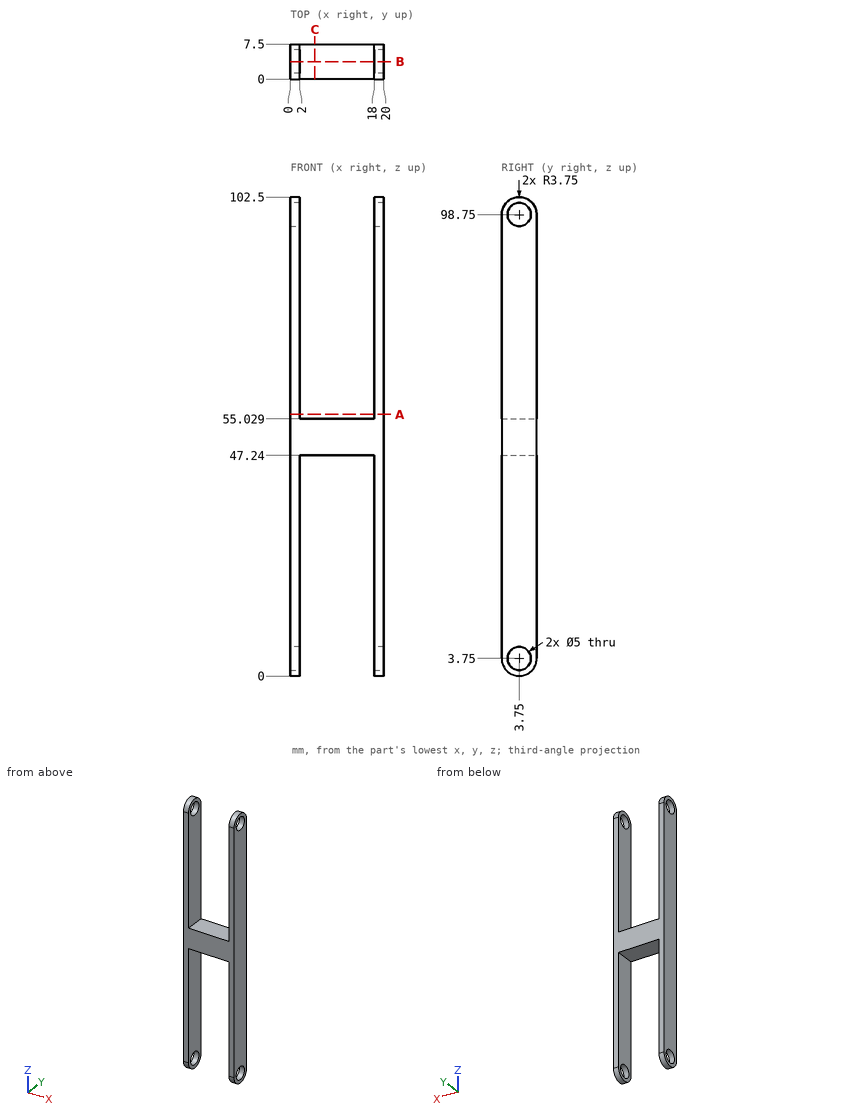
Study the drawing (mm; zero at the part's minimum x, y, z) and answer. Round coordinates to 2 decimals unless told otherwise and drop trailing zeros. Write each loop counter-clockwise with the first axis right and the second up, starting at its lowest first coordinate (ties: lowest second). Pieces come first, ordered by that corner, then holes.
Q1. Find section A-A on z = 56. Determine the outline of the cut face in (x, y).
Values:
outline: (0, 0) - (2, 0) - (2, 7.5) - (0, 7.5) - close; (18, 0) - (20, 0) - (20, 7.5) - (18, 7.5) - close
Q2. Find section C-C on x = 5.25. Determine the outline of the cut face in (y, z), and give its area (3 significant figures).
Values:
outline: (0, 47.24) - (7.5, 47.24) - (7.5, 55.03) - (0, 55.03) - close
area: 58.4 mm2
Q3. A flat-ended cylindrical pin translates along its axis: P1, Ø5, axis at x = 14, z = 75, coming from the +Y side. Find the tip coordinate at first contact, or state that the pin passes through.
Values:
P1: passes through
Q4. Straight lines are drawn through the part: line 1 (Z direction, x = 1, y = 4.5) (1 decimal); line 2 (Y direction, x = 0.85, z = 3.75); line 3 (X direction, y = 6.5, z = 82). For each, find the intervals that lie inside material, in ascending order.
Values:
line 1: z = 0.1 to 1.4, 6.1 to 96.4, 101.1 to 102.4
line 2: y = 0 to 1.25, 6.25 to 7.5
line 3: x = 0 to 2, 18 to 20
Q5. Find section B-B on y = 3.75. Determine the outline of the cut face in (x, z).
Values:
outline: (0, 0) - (2, 0) - (2, 1.25) - (0, 1.25) - close; (0, 6.25) - (2, 6.25) - (2, 47.24) - (18, 47.24) - (18, 6.25) - (20, 6.25) - (20, 96.25) - (18, 96.25) - (18, 55.03) - (2, 55.03) - (2, 96.25) - (0, 96.25) - close; (0, 101.25) - (2, 101.25) - (2, 102.5) - (0, 102.5) - close; (18, 0) - (20, 0) - (20, 1.25) - (18, 1.25) - close; (18, 101.25) - (20, 101.25) - (20, 102.5) - (18, 102.5) - close
